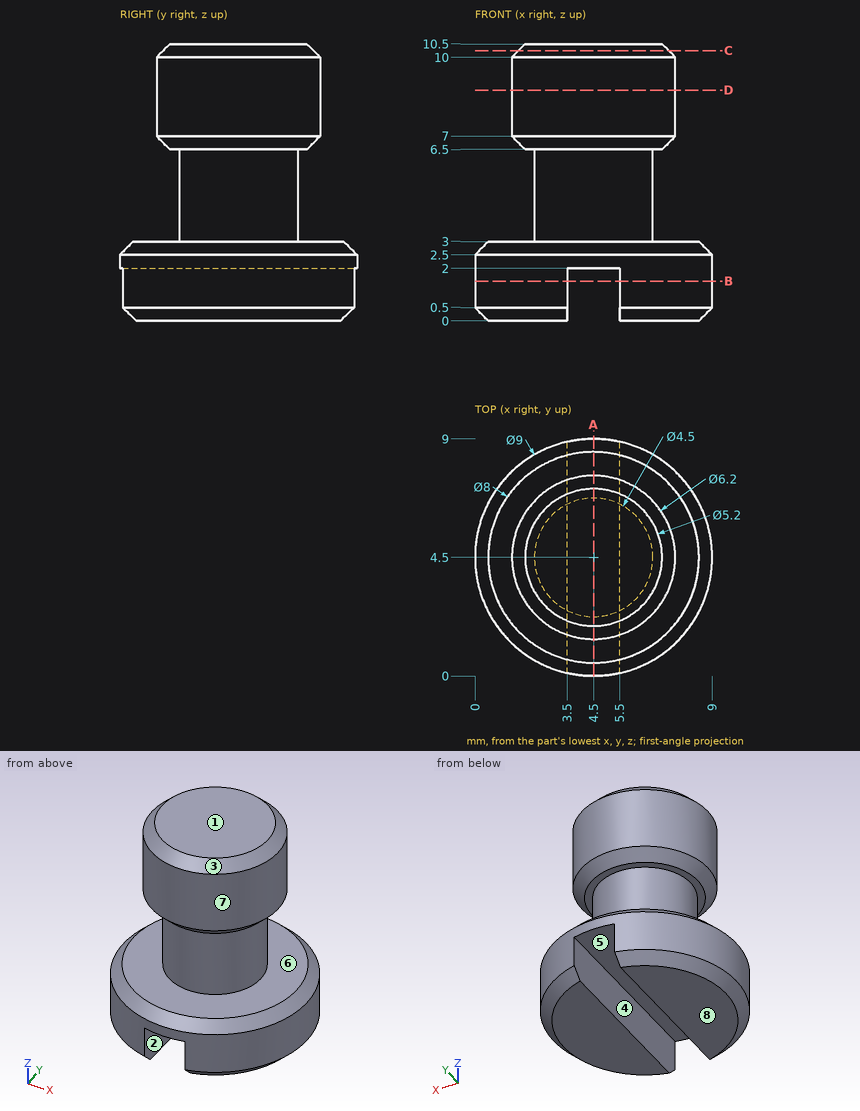
Input: dimensioned drawing with shaded views. Units: mm. Origin: part minimum x, y, z. A direction names the side the tool comes from. Give positions to 0.01 mm unless a question says otherwise; leave off trailing zeros. Order: outer loops, then holes, each group sorted by start corner. A loop starts at its lowest first (then second) coordinate and runs counter-clockwise, first axis right, second up. Notation, with made-up numbers: (-38, -12) -> (-22, -12) arc R20 cw to (-22, 16) -> close; hole circle Ø1 at (12, 62.25). An arc over 180 degrees is marked (long way). Use one line per item in the form item = value.
1) Reachability of the marked faces 5, 6, 7 and 8 from +Z, -Z, +X, -X, +Y, -Y: full face, straight path, thin tool, end or side. Return the list, or none.
Response values:
face_5 = -Z, +Y, -Y
face_6 = none
face_7 = +Z
face_8 = -Z, +X, -X, +Y, -Y
2) Mould query, pull axis X, two halves, no side actions, for the marked faces 1, 2, 3 and 4. Classes: pulls with the +X half, pulls with the -X half, needs draft (parallel to the pull), parting line crosses it, or undercut.
Response values:
face_1 = needs draft
face_2 = undercut
face_3 = parting line crosses it
face_4 = undercut
3) Section C-C, the plane z = 10.25. Return loops of the section in (x, y).
Response values:
outline = circle Ø5.7 at (4.5, 4.5)
4) Section B-B, the plane z = 1.5. Return loops of the section in (x, y), and give its area (3 significant figures).
Response values:
outline = (3.5, 0.11) -> (3.5, 8.89) arc R4.5 ccw to start; (5.5, 0.11) arc R4.5 ccw to (5.5, 8.89) -> close
area = 45.8 mm^2
5) Line query: probe 1 along Z at (x, y) = (5.75, 7); probe 2 along Z at (x, y) = (4.5, 5); probe 3 along Z at (x, y) = (4, 1.75). Output: solid intervals per line, ascending.
Response values:
probe_1 = 0 to 3, 6.7 to 10.3
probe_2 = 2 to 10.5
probe_3 = 2 to 3, 6.7 to 10.3
6) First-contact query: pin 1 Ø1.6 at (y, z) = (2.5, 1) entering from +X; pin 2 Ø1 at (y, z) = (6, 1) entering from -X; pin 3 Ø5 at (y, z) = (3, 5) entering from -X. Flat tips, straight axial feed; report the tip coordinate or a pass-through.
Response values:
pin_1 = 8.84
pin_2 = 0.11
pin_3 = 0.16
7) Section A-A, the plane x = 4.5. Return loops of the section in (y, z).
Response values:
outline = (0, 2) -> (9, 2) -> (9, 2.5) -> (8.5, 3) -> (6.75, 3) -> (6.75, 6.5) -> (7.1, 6.5) -> (7.6, 7) -> (7.6, 10) -> (7.1, 10.5) -> (1.9, 10.5) -> (1.4, 10) -> (1.4, 7) -> (1.9, 6.5) -> (2.25, 6.5) -> (2.25, 3) -> (0.5, 3) -> (0, 2.5) -> close
8) Section D-D, the plane z = 8.75. Return loops of the section in (x, y), and give its area (3 significant figures).
Response values:
outline = circle Ø6.2 at (4.5, 4.5)
area = 30.2 mm^2
